```python
from build123d import *

# Parameters (mm, degrees)
SKETCH1_W           = 12.7
SKETCH1_H           = 12.7
BOSS_EXTRUDE1_DEPTH = 25.4
SKETCH2_R           = 3.175
CUT_EXTRUDE1_DEPTH  = 30.099355663
SKETCH4_R           = 3.175
CUT_EXTRUDE2_DEPTH  = 30.099355663


with BuildPart() as part:
    # Sketch1 → Boss-Extrude1 (new, symmetric)
    with BuildSketch(Plane.XY):
        Rectangle(SKETCH1_W, SKETCH1_H)
    extrude(amount=BOSS_EXTRUDE1_DEPTH, both=True)

    # Sketch2 → Cut-Extrude1 (cut, through all)
    with BuildSketch(Plane(origin=(0, 6.35, 0), x_dir=(1, 0, 0), z_dir=(0, 1, 0))):
        with Locations(Location((0, 19.05, 0), (0, 0, 270))):
            Circle(SKETCH2_R)
        with Locations(Location((0, 6.35, 0), (0, 0, 270))):
            Circle(SKETCH2_R)
        with Locations(Location((0, -6.35, 0), (0, 0, 270))):
            Circle(SKETCH2_R)
        with Locations(Location((0, -19.05, 0), (0, 0, 270))):
            Circle(SKETCH2_R)
        with Locations((0, -31.75)):
            Circle(SKETCH2_R)
        with Locations((0, -44.45)):
            Circle(SKETCH2_R)
    extrude(amount=-CUT_EXTRUDE1_DEPTH, mode=Mode.SUBTRACT)

    # Sketch4 → Cut-Extrude2 (cut, through all)
    with BuildSketch(Plane.ZY.offset(6.35)):
        with Locations((19.05, 0)):
            Circle(SKETCH4_R)
        with Locations((6.35, 0)):
            Circle(SKETCH4_R)
        with Locations((-6.35, 0)):
            Circle(SKETCH4_R)
        with Locations((-19.05, 0)):
            Circle(SKETCH4_R)
        with Locations((-31.75, 0)):
            Circle(SKETCH4_R)
        with Locations((-44.45, 0)):
            Circle(SKETCH4_R)
    extrude(amount=-CUT_EXTRUDE2_DEPTH, mode=Mode.SUBTRACT)


solid = part.part
```
Work out the finished part from the listing and answer in its coordinate system (mm). Coordinates: 2 decimals unless noted, no trailing zeros. Loops run counter-clockwise (first coordinate to the right, second up) from the corner with the lowest first, then second, coordinate; pieces in that order, holes last. Notation, with made-up numbers: (14, 4) - (29, 4) arc R12 ccw to (29, 9) - close; hole circle Ø8 at (72.25, -15.75). An arc over 180 degrees is marked (long way). Use a Markdown table: item, result.
Item 1: Consider probe 1 along Z at (x, y) = (-1.75, 0) (3 decimals); probe 2 along X at (y, z) = (5.25, -19); probe 3 along Y at (x, z) = (3.5, 19.05) (3 decimals). Determine where each line is inside the solid, lowest interval first. Write a range as from..to.
Evaluation:
| item | result |
|---|---|
| probe 1 | z = -25.4..-22.225, -15.875..-9.525, -3.175..3.175, 9.525..15.875, 22.225..25.4 |
| probe 2 | x = -6.35..-3.17, 3.17..6.35 |
| probe 3 | y = -6.35..-3.175, 3.175..6.35 |
Item 2: The mould has two halves that part along X. Classify faces 1 (the flat face through (0, 0, 25.4)), 2 (the cylindrical face through (2.146, 3.925, 16.71)), 3 (the flat face through (6.35, 0, 0)): +X half, -X half, draft (parallel to the pull), parting line (faces both ways), or undercut.
Evaluation:
| item | result |
|---|---|
| face 1 | draft |
| face 2 | undercut |
| face 3 | +X half |
Item 3: Find section A-A, the plane z = 6.35. Determine the outline of the cut face in (x, y) (3 decimals).
Evaluation:
| item | result |
|---|---|
| outline | (-6.35, -6.35) - (-3.175, -6.35) - (-3.175, -3.175) - (-6.35, -3.175) - close; (-6.35, 3.175) - (-3.175, 3.175) - (-3.175, 6.35) - (-6.35, 6.35) - close; (3.175, -6.35) - (6.35, -6.35) - (6.35, -3.175) - (3.175, -3.175) - close; (3.175, 3.175) - (6.35, 3.175) - (6.35, 6.35) - (3.175, 6.35) - close |
Item 4: Find section B-B, the plane y = -3.75. Determine the outline of the cut face in (x, z) (3 decimals), and give its area (3 significant figures).
Evaluation:
| item | result |
|---|---|
| outline | (-6.35, -25.4) - (6.35, -25.4) - (6.35, 25.4) - (-6.35, 25.4) - close; hole circle Ø6.35 at (0, -19.05); hole circle Ø6.35 at (0, -6.35); hole circle Ø6.35 at (0, 6.35); hole circle Ø6.35 at (0, 19.05) |
| area | 518 mm2 |
Item 5: Find section D-D, the plane x = -1. State how many separate pieces and enclosed holes the cut face has, and give its area (3 significant figures).
Evaluation:
| item | result |
|---|---|
| separate pieces | 5 |
| enclosed holes | 0 |
| area | 337 mm2 |
